Input: part model. Units: mm. Frame: model coordinates. A direction names the side the tool comes from. Give positions to 0.01 mm unless a question says otherwise; leave off trailing zeros. Order: outer loops, then holes, each group sorted by start corner. A loop starts at its lowest first (then second) coordinate and runs counter-clockwise, first axis right, second up. Notation, with made-up numbers: (-7.75, 32) - (9.25, 32) arc R14 cw to (9.25, 48) - close; hole circle Ø2 at (12, -4.75). An arc over 180 degrees is marked (long way). Answer in a Markdown table with one row per item. Add a question column.
from build123d import *

# Parameters (mm, degrees)
SKETCH1_R               = 17.5
SKETCH1_R_2             = 12
BOSS_EXTRUDE1_DEPTH     = 21
SKETCH1_3_R             = 31.5
SKETCH1_3_R_2           = 26
BOSS_EXTRUDE2_DEPTH     = 35
SKETCH1_4_R             = 31.5
SKETCH1_4_R_2           = 5
BOSS_EXTRUDE3_DEPTH     = 21
BOSS_EXTRUDE4_DEPTH     = 2.5
CUT_EXTRUDE1_DEPTH      = 311.166315701
CUT_EXTRUDE1_DEPTH_BACK = 311.166315701
SKETCH1_6_R             = 17.5
SKETCH1_6_R_2           = 12
BOSS_EXTRUDE5_DEPTH     = 21
SKETCH1_7_R             = 5
CUT_EXTRUDE2_DEPTH      = 14


with BuildPart() as part:
    # Sketch1 → Boss-Extrude1 (new, symmetric)
    with BuildSketch(Plane(origin=(0, 0, 0), x_dir=(1, 0, 0), z_dir=(0, 1, 0))):
        with Locations(Location((0, 0, 0), (0, 0, 90))):
            Circle(SKETCH1_R)
        with Locations(Location((0, 0, 0), (0, 0, 90))):
            Circle(SKETCH1_R_2, mode=Mode.SUBTRACT)
    extrude(amount=BOSS_EXTRUDE1_DEPTH, both=True)



with BuildPart() as body_2:
    # Sketch1_3 → Boss-Extrude2 (new, symmetric)
    with BuildSketch(Plane(origin=(0, 0, 0), x_dir=(1, 0, 0), z_dir=(0, 1, 0))):
        with Locations(Location((-250, 0, 0), (0, 0, 270))):
            Circle(SKETCH1_3_R)
        with Locations(Location((-250, 0, 0), (0, 0, 270))):
            Circle(SKETCH1_3_R_2, mode=Mode.SUBTRACT)
    extrude(amount=BOSS_EXTRUDE2_DEPTH, both=True)


with BuildPart() as part_1:
    add(part.part)

    add(body_2.part)  # Boss-Extrude3 merges body 2
    # Sketch1_4 → Boss-Extrude3 (add, symmetric)
    with BuildSketch(Plane(origin=(0, 0, 0), x_dir=(1, 0, 0), z_dir=(0, 1, 0))):
        with BuildLine():
            ThreePointArc((-10.131953212, 14.268620259), (-20.198477773, 9.324322534), (-31.312052828, 7.817854403))
            Line((-31.312052828, 7.817854403), (-162, 11.240038738))
            ThreePointArc((-162, 11.240038738), (-197.875878659, 21.911731191), (-223.547039722, 49.150585409))
            ThreePointArc((-223.547039722, 49.150585409), (-227.777941589, 53.8093419), (-233.701306889, 55.934967963))
            ThreePointArc((-233.701306889, 55.934967963), (-271.66540115, 49.388348587), (-300.819950957, 24.206154404))
            ThreePointArc((-300.819950957, 24.206154404), (-302.758398561, 19.494647504), (-302.737346662, 14.4))
            ThreePointArc((-302.737346662, 14.4), (-301.282651255, 0), (-302.737346662, -14.4))
            ThreePointArc((-302.737346662, -14.4), (-302.758398561, -19.494647504), (-300.819950957, -24.206154404))
            ThreePointArc((-300.819950957, -24.206154404), (-271.66540115, -49.388348587), (-233.701306889, -55.934967963))
            ThreePointArc((-233.701306889, -55.934967963), (-227.777941589, -53.8093419), (-223.547039722, -49.150585409))
            ThreePointArc((-223.547039722, -49.150585409), (-197.875878659, -21.911731191), (-162, -11.240038738))
            Line((-162, -11.240038738), (-31.312052828, -7.817854403))
            ThreePointArc((-31.312052828, -7.817854403), (-20.198477773, -9.324322534), (-10.131953212, -14.268620259))
            ThreePointArc((-10.131953212, -14.268620259), (-17.5, 0), (-10.131953212, 14.268620259))
        make_face()
        with Locations(Location((-250, 0, 0), (0, 0, 270))):
            Circle(SKETCH1_4_R, mode=Mode.SUBTRACT)
        with BuildLine():
            ThreePointArc((-180, -6), (-186, 0), (-180, 6))
            Line((-180, 6), (-30, 6))
            ThreePointArc((-30, 6), (-24, 0), (-30, -6))
            Line((-30, -6), (-180, -6))
        make_face(mode=Mode.SUBTRACT)
        with Locations(Location((-290, 17, 0), (0, 0, 90))):
            Circle(SKETCH1_4_R_2, mode=Mode.SUBTRACT)
        with Locations(Location((-235, 43, 0), (0, 0, 90))):
            Circle(SKETCH1_4_R_2, mode=Mode.SUBTRACT)
        with Locations(Location((-235, -43, 0), (0, 0, 90))):
            Circle(SKETCH1_4_R_2, mode=Mode.SUBTRACT)
        with Locations(Location((-290, -17, 0), (0, 0, 90))):
            Circle(SKETCH1_4_R_2, mode=Mode.SUBTRACT)
    extrude(amount=BOSS_EXTRUDE3_DEPTH, both=True)

    # Sketch1_5 → Boss-Extrude4 (add, symmetric)
    with BuildSketch(Plane(origin=(0, 0, 0), x_dir=(1, 0, 0), z_dir=(0, 1, 0))):
        with BuildLine():
            Line((-180, -6), (-30, -6))
            ThreePointArc((-30, -6), (-24, 0), (-30, 6))
            Line((-30, 6), (-180, 6))
            ThreePointArc((-180, 6), (-186, 0), (-180, -6))
        make_face()
    extrude(amount=BOSS_EXTRUDE4_DEPTH, both=True)

    # Sketch3 → Cut-Extrude1 (cut, two sides: drawn at the far end of the back side and taken through both)
    with BuildSketch(Plane.XY.offset(-CUT_EXTRUDE1_DEPTH_BACK)):
        with BuildLine():
            ThreePointArc((-162, -21), (-145.170802033, -14.478720031), (-127.293303783, -12))
            Line((-127.293303783, -12), (17.5, -8.840598872))
            Line((17.5, -8.840598872), (17.5, -21))
            Line((17.5, -21), (-162, -21))
        make_face()
        with BuildLine():
            Line((-162, 21), (17.5, 21))
            Line((17.5, 21), (17.5, 8.840598872))
            Line((17.5, 8.840598872), (-127.293303783, 12))
            ThreePointArc((-127.293303783, 12), (-145.170802033, 14.478720031), (-162, 21))
        make_face()
    extrude(amount=CUT_EXTRUDE1_DEPTH + CUT_EXTRUDE1_DEPTH_BACK, mode=Mode.SUBTRACT)

    # Sketch1_6 → Boss-Extrude5 (add, symmetric)
    with BuildSketch(Plane(origin=(0, 0, 0), x_dir=(1, 0, 0), z_dir=(0, 1, 0))):
        with Locations(Location((0, 0, 0), (0, 0, 270))):
            Circle(SKETCH1_6_R)
        with Locations(Location((0, 0, 0), (0, 0, 90))):
            Circle(SKETCH1_6_R_2, mode=Mode.SUBTRACT)
    extrude(amount=BOSS_EXTRUDE5_DEPTH, both=True)

    # Sketch1_7 → Cut-Extrude2 (cut, symmetric)
    with BuildSketch(Plane(origin=(0, 0, 0), x_dir=(1, 0, 0), z_dir=(0, 1, 0))):
        with BuildLine():
            ThreePointArc((-231.201580847, 25.275866699), (-198.167794768, 10.53206878), (-162, 11.240038738))
            ThreePointArc((-162, 11.240038738), (-197.875878659, 21.911731191), (-223.547039722, 49.150585409))
            ThreePointArc((-223.547039722, 49.150585409), (-227.777941589, 53.8093419), (-233.701306889, 55.934967963))
            ThreePointArc((-233.701306889, 55.934967963), (-271.66540115, 49.388348587), (-300.819950957, 24.206154404))
            ThreePointArc((-300.819950957, 24.206154404), (-302.758398561, 19.494647504), (-302.737346662, 14.4))
            ThreePointArc((-302.737346662, 14.4), (-301.282651255, 0), (-302.737346662, -14.4))
            ThreePointArc((-302.737346662, -14.4), (-302.758398561, -19.494647504), (-300.819950957, -24.206154404))
            ThreePointArc((-300.819950957, -24.206154404), (-271.66540115, -49.388348587), (-233.701306889, -55.934967963))
            ThreePointArc((-233.701306889, -55.934967963), (-227.777941589, -53.8093419), (-223.547039722, -49.150585409))
            ThreePointArc((-223.547039722, -49.150585409), (-197.875878659, -21.911731191), (-162, -11.240038738))
            ThreePointArc((-162, -11.240038738), (-198.167794768, -10.53206878), (-231.201580847, -25.275866699))
            ThreePointArc((-231.201580847, -25.275866699), (-281.5, 0), (-231.201580847, 25.275866699))
        make_face()
        with Locations(Location((-235, -43, 0), (0, 0, 90))):
            Circle(SKETCH1_7_R, mode=Mode.SUBTRACT)
        with Locations(Location((-290, -17, 0), (0, 0, 90))):
            Circle(SKETCH1_7_R, mode=Mode.SUBTRACT)
        with Locations(Location((-290, 17, 0), (0, 0, 90))):
            Circle(SKETCH1_7_R, mode=Mode.SUBTRACT)
        with Locations(Location((-235, 43, 0), (0, 0, 90))):
            Circle(SKETCH1_7_R, mode=Mode.SUBTRACT)
    extrude(amount=CUT_EXTRUDE2_DEPTH, both=True, mode=Mode.SUBTRACT)


solid = part_1.part
Q1. Access query for faces 4 (the flat face through (-121, -8, 6)), 5 (the cylindrical face through (-198.668, 0.196, -10.635)), 6 (the flat face through (-218, 21, -1)), 7 (the cylindrical face through (-144.926, 14.416, -8.657)). Directions: +Z, -Z, +X, -X, +Y, -Y. A direction counts if a zero-diameter tool reaches every point of the face in a straight line with its end or side. Return the directions, or none.
Q2. Section C-C, the plane x = -270. Return loops of the section in (y, z).
Q3. Section A-A, the plane y = 17. Return loops of the section in (x, z).
Q4. Section D-D, the plane x = -201. Return loops of the section in (y, z).
Q5. Section B-B, the plane z = 44. Return loops of the section in (x, y).
Q6. Pull-direction query (Z, two-part tool) for faces 1 (the cylindrical face through (-272.158, -17.451, 49.153)), 2 (the cylindrical face through (-271.17, -17.45, -49.62)), 3 (the cylindrical face through (-275.38, -0.49, -5.64)); classes: +Z half, -Z half, draft (parallel to the pull), parting line (faces both ways), or undercut.
Q7. Contact query for flat-ended pins moving along their axis: P1, Ø8, axis at x = -238, z = -43.5, coming from the -Y side; P2, Ø9, axis at x = -106.5, y = 10, coming from the +Z side; P3, Ø13, axis at x = -290, z = -17, coming from the +Y side; P4, Ø21.5, axis at x = 0, z = 0, coming from the -Y side. Output: stop coordinate, or through.
Q8. Line query: probe 1 along X at (y, z) = (-12.5, 0); probe 2 along X at (y, z) = (-18, 0); probe 3 along Z at (x, y) = (-290, 16.5). Output: solid intervals per line, ascending.
Computed:
| question | item | result |
|---|---|---|
| 1 | face 4 | -Y |
| 1 | face 5 | -Z |
| 1 | face 6 | +Y |
| 1 | face 7 | +Z, -Z, +Y |
| 2 | outline | (-35, -24.34) - (-21, -24.34) - (-21, -50.15) - (-14, -50.15) - (-14, -24.34) - (14, -24.34) - (14, -50.15) - (21, -50.15) - (21, -24.34) - (35, -24.34) - (35, -16.61) - (-35, -16.61) - close; (-35, 16.61) - (35, 16.61) - (35, 24.34) - (21, 24.34) - (21, 50.15) - (14, 50.15) - (14, 24.34) - (-14, 24.34) - (-14, 50.15) - (-21, 50.15) - (-21, 24.34) - (-35, 24.34) - close |
| 3 | outline | (-302.74, -14.4) arc R13 ccw to (-300.82, -24.21) arc R72 ccw to (-233.7, -55.93) arc R13 ccw to (-223.55, -49.15) arc R72 cw to (-162, -11.24) - (-153.12, -11.01) - (-153.12, -6) - (-180, -6) arc R6 cw to (-180, 6) - (-153.12, 6) - (-153.12, 11.01) - (-162, 11.24) arc R72 cw to (-223.55, 49.15) arc R13 ccw to (-233.7, 55.93) arc R72 ccw to (-300.82, 24.21) arc R13 ccw to (-302.74, 14.4) arc R72 cw to start; circle Ø35 at (0, 0); hole circle Ø10 at (-290, -17); hole circle Ø10 at (-290, 17); hole circle Ø52 at (-250, 0); hole circle Ø10 at (-235, -43); hole circle Ø10 at (-235, 43); hole circle Ø24 at (0, 0) |
| 4 | outline | (-21, -23.95) - (-14, -23.95) - (-14, -11.16) - (14, -11.16) - (14, -23.95) - (21, -23.95) - (21, 23.95) - (14, 23.95) - (14, 11.16) - (-14, 11.16) - (-14, 23.95) - (-21, 23.95) - close |
| 5 | outline | (-281.13, -21) - (-239.9, -21) - (-239.9, -14) - (-281.13, -14) - close; (-281.13, 14) - (-239.9, 14) - (-239.9, 21) - (-281.13, 21) - close; (-230.1, -21) - (-220.5, -21) - (-220.5, -14) - (-230.1, -14) - close; (-230.1, 14) - (-220.5, 14) - (-220.5, 21) - (-230.1, 21) - close |
| 6 | face 1 | +Z half |
| 6 | face 2 | -Z half |
| 6 | face 3 | undercut |
| 7 | P1 | stops at y = -21 |
| 7 | P2 | stops at z = 9.9 |
| 7 | P3 | stops at y = 21 |
| 7 | P4 | passes through |
| 8 | probe 1 | x = -281.5 to -276, -224 to -186, -17.5 to -12, 12 to 17.5 |
| 8 | probe 2 | x = -301.28 to -276, -224 to -186, -17.5 to -12, 12 to 17.5 |
| 8 | probe 3 | z = -36.95 to -22, -12 to 12, 22 to 36.95 |
